Work out the finished part from the listing and answer in its coordinate system (mm). Round coordinates to 2 decimals unless told otherwise and drop trailing zeros. Use a Markdown table: item, result. Add a question column.
Item 1: A cutting plane is placed at A-A, the plane y = -5.25. Give the number of separate pieces and of enclosed holes in the cut face, plus the area to 3 significant figures.
Item 2: Find the intervals of material crossed by L1, parallel to Z at x = 108.5, y = -7; L2, parallel to X at y = -2.25, z = 44; L3, parallel to Z at x = -113.5, y = -2, in increasing order. Write a range as [from, to].
Item 3: Flat-ended cylindrical pins translate along their axes: P1, Ø24.5, axis at x = 106.25, z = 44.01, coming from the -Y side; P2, Ø5, axis at x = 12, y = -15, coming from the +Z side; P3, Ø3, axis at y = -4, z = -105.5, coming from the -X side; P4, Ø4, axis at x = 25.5, y = -15, coming from the +Z side. Find the tip coordinate at first contact, or state that the pin passes through.
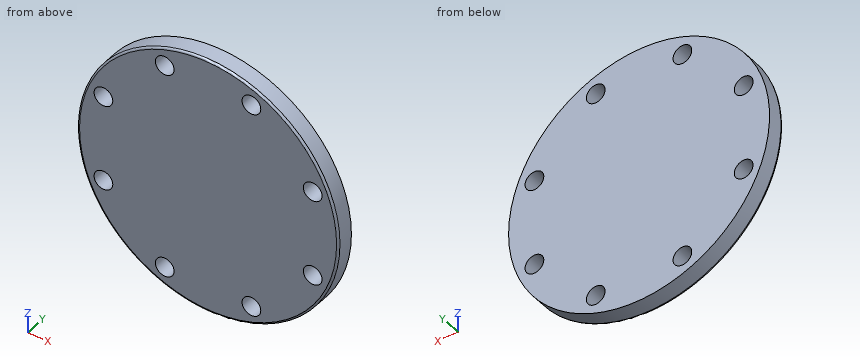
from build123d import *

# Parameters (mm, degrees)
F0_R     = 132.5
F0_R_2   = 9.5
F1_DEPTH = 18
F2_R     = 2


with BuildPart() as f1:
    # F0 (on Front) → F1 (new body)
    with BuildSketch(Plane.XZ):
        Circle(F0_R)
        with Locations((-44.008595, -106.246146)):
            Circle(F0_R_2, mode=Mode.SUBTRACT)
        with Locations((-106.246146, -44.008595)):
            Circle(F0_R_2, mode=Mode.SUBTRACT)
        with Locations((44.008595, -106.246146)):
            Circle(F0_R_2, mode=Mode.SUBTRACT)
        with Locations((106.246146, -44.008595)):
            Circle(F0_R_2, mode=Mode.SUBTRACT)
        with Locations((-106.246146, 44.008595)):
            Circle(F0_R_2, mode=Mode.SUBTRACT)
        with Locations((-44.008595, 106.246146)):
            Circle(F0_R_2, mode=Mode.SUBTRACT)
        with Locations((106.246146, 44.008595)):
            Circle(F0_R_2, mode=Mode.SUBTRACT)
        with Locations((44.008595, 106.246146)):
            Circle(F0_R_2, mode=Mode.SUBTRACT)
    extrude(amount=F1_DEPTH)

    # F2
    f2_edges = [f1.edges().sort_by_distance(p)[0] for p in [
        (-132.5, -18, 0),
    ]]
    fillet(f2_edges, radius=F2_R)


solid = f1.part
Reported:
| question | item | result |
|---|---|---|
| 1 | separate pieces | 1 |
| 1 | enclosed holes | 8 |
| 1 | area | 52,900 mm² |
| 2 | L1 | [-76.05, -53.24], [-34.78, 34.78], [53.24, 76.05] |
| 2 | L2 | [-124.98, -115.75], [-96.75, 96.75], [115.75, 124.98] |
| 2 | L3 | [-68.37, -50.14], [-37.87, 37.87], [50.14, 68.37] |
| 3 | P1 | y = -18 |
| 3 | P2 | z = 132.16 |
| 3 | P3 | x = -82.1 |
| 3 | P4 | z = 130.4 |
